Study the drawing (mm; zero at the part's minimum x, y, z) and answer. A direction names the side the tool comes from. Round coordinates to 2 decimals unless told otherwise and drop trailing zeros. Loops run counter-clockwise (first coordinate to the right, second up) from the corner with the lowest first, then second, coordinate; pieces in that order, holes last. Notation, with made-up numbers: (43, 15.5) - (101, 15.5) arc R19 cw to (101, 35.5) - close; hole circle Ø9 at (-30, 29). An arc over 180 degrees is marked (long way). Use CSV: the item, a comma, the result in double quotes. Start each with the question number.
1. Consider line 1 along Y through (x, z) = (4.5, 2.9); line 2 along Z through (x, y) = (21.5, 7.5); line 3 along Y through (x, z) = (21, 10.25). Determine where each line is inside the solid, lowest interval first.
2. A tool of negligible diameter and unlimited length cuts with its end or side. For the marked faces 1 and 2, from which of +Z, -Z, +X, -X, +Y, -Y can it reach the whole face along a straight path? Write none if from no direction.
3. Find section B-B (z = 3.25). Give the vertices of the cut face in (x, y), and give its area (3 significant figures).
4. Find section C-C (x = 37.5). Give the vertices of the cut face in (y, z).
5. Determine the mould class of the marked faces 3, 4, 5 and 6 for opening direction Y: +Y half, -Y half, draft (parallel to the pull), parting line (faces both ways), or undercut.
6. Find section A-A (y = 37.5). Give the vertices of the cut face in (x, z).
7. Given pin 1 Ø6 at (x, y) = (7.5, 15.5) entering from +Z; pin 2 Ø1.5 at (y, z) = (24, 9.5) entering from +X; pin 3 Ø8 at (y, z) = (12.5, 11.5) entering from -X, each flat-ended and moving along its own axis, determine where each tip first touches the part or whether it passes through.
8. Find section D-D (y = 4.5). Give the vertices of the cut face in (x, z).
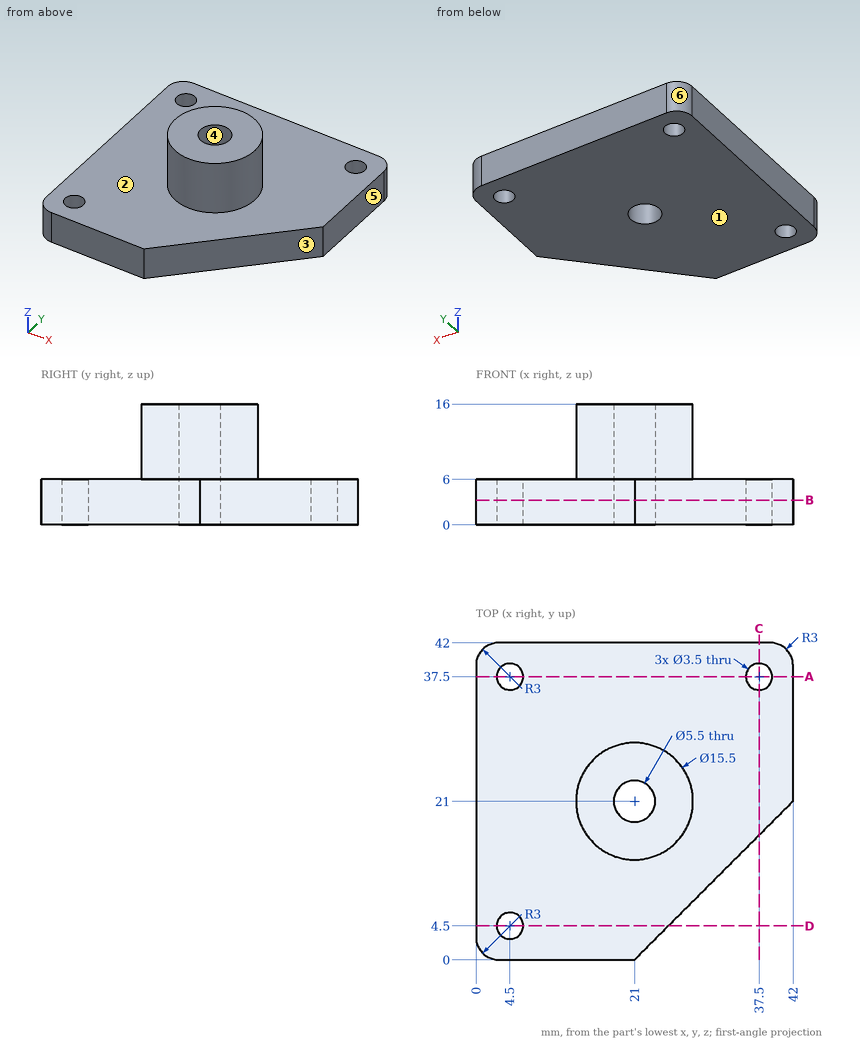
Filled sheet:
1,line 1,"y = 0 to 2.75, 6.25 to 35.75, 39.25 to 42"
1,line 2,"z = 0 to 6"
1,line 3,"y = 13.25 to 18.25, 23.75 to 28.75"
2,face 1,"-Z, +X, -X, +Y, -Y"
2,face 2,"+Z"
3,outline,"(0, 3) arc R3 ccw to (3, 0) - (21, 0) - (42, 21) - (42, 39) arc R3 ccw to (39, 42) - (3, 42) arc R3 ccw to (0, 39) - close; hole circle Ø3.5 at (4.5, 4.5); hole circle Ø3.5 at (4.5, 37.5); hole circle Ø5.5 at (21, 21); hole circle Ø3.5 at (37.5, 37.5)"
3,area,"1,490 mm²"
4,outline,"(16.5, 0) - (35.75, 0) - (35.75, 6) - (16.5, 6) - close; (39.25, 0) - (42, 0) - (42, 6) - (39.25, 6) - close"
5,face 3,"-Y half"
5,face 4,"undercut"
5,face 5,"draft"
5,face 6,"+Y half"
6,outline,"(0, 0) - (2.75, 0) - (2.75, 6) - (0, 6) - close; (6.25, 0) - (35.75, 0) - (35.75, 6) - (6.25, 6) - close; (39.25, 0) - (42, 0) - (42, 6) - (39.25, 6) - close"
7,pin 1,"stops at z = 6"
7,pin 2,"stops at x = 28.42"
7,pin 3,"stops at x = 14.69"
8,outline,"(0, 0) - (2.75, 0) - (2.75, 6) - (0, 6) - close; (6.25, 0) - (25.5, 0) - (25.5, 6) - (6.25, 6) - close"
